Source: CAD feature listing. Evaluate the final solid. Frame: model axes, mm. A direction names the side the tool comes from. Give positions to 0.01 mm unless a question says otherwise; leave off trailing zeros. Loops run counter-clockwise (first coordinate to the right, second up) from the corner with the lowest first, then second, coordinate; pieces in that order, holes last. Notation, with made-up numbers: (-24, 88) -> (27, 88) arc R14 cw to (27, 97) -> close; hole circle Ø11 at (14, 10). An arc over 180 degrees is marked (long way). Put each result on its own line as item: value.
```python
from build123d import *

# Parameters (mm, degrees)
F0_W      = 13.86
F0_H      = 7.73
F1_DEPTH  = 2.14
F3_DEPTH  = 13.861
F4_W      = 1.7220231239
F4_H      = 4.1921688244
F5_DEPTH  = 1.48
F6_R      = 3.43
F7_DEPTH  = 1.48
F8_R      = 1.14
F10_DEPTH = 3.34
F9_R      = 1.1457110781
F11_DEPTH = 3.34
F12_R     = 1.54
F13_DEPTH = 4.39


with BuildPart() as f1:
    # F0 (on Front) → F1 (new body)
    with BuildSketch(Plane.XZ):
        with Locations((0.6576154042, 6.5625002608)):
            Rectangle(F0_W, F0_H)
    extrude(amount=F1_DEPTH)

    # F2 (on face) → F3 (cut, through all)
    with BuildSketch(Plane.YZ.offset(7.5876154042)):
        with BuildLine():
            add(Edge.make_bspline(
                [(-2.14, 4.4675002608), (-1.0178836739, 5.1285764004), (-1.0178836739, 10.7190171735), (-7.3584975292, 6.5625002608), (-3.2052818458, 3.8399072084), (-2.14, 4.4675002608)],
                knots=[0, 0, 0, 0, 0.3449820825, 0.6724910412, 1, 1, 1, 1], degree=3))
        make_face()
    extrude(amount=-F3_DEPTH, mode=Mode.SUBTRACT)

    # F4 (on Right) → F5 (join)
    with BuildSketch(Plane.YZ):
        with Locations((-2.9032976599, 6.5771206282)):
            Rectangle(F4_W, F4_H)
        Polygon((-2.042286098, 8.6732050404), (-2.042286098, 4.481036216), (-1.0486273095, 4.481036216), (-1.0486273095, 8.7523022667), align=None)
    extrude(amount=F5_DEPTH)

    # F6 (on face) → F7 (join)
    with BuildSketch(Plane.YZ.offset(1.48)):
        with Locations((-5.5470176696, 6.5771206282)):
            Circle(F6_R)
    extrude(amount=-F7_DEPTH)

    # F8 (on face) → F10 (join)
    with BuildSketch(Plane.YZ.offset(1.48)):
        with Locations((-5.5470176696, 6.5771206282)):
            Circle(F8_R)
    extrude(amount=F10_DEPTH)

    # F9 (on face) → F11 (join)
    with BuildSketch(Plane(origin=(0, 0, 0), x_dir=(0, -1, 0), z_dir=(-1, 0, 0))):
        with Locations((5.5470176696, 6.5771206282)):
            Circle(F9_R)
    extrude(amount=F11_DEPTH)

    # F12 (on face) → F13 (join)
    with BuildSketch(Plane(origin=(0, 0, 0), x_dir=(-1, 0, 0), z_dir=(0, 1, 0))):
        Polygon((-1.8146777797, 7.6139823431), (-3.245869735, 9.0531328988), (-5.2755083889, 9.0587604791), (-6.7146589446, 7.6275685238), (-6.7202865249, 5.59792987), (-5.2890945696, 4.1587793143), (-3.2594559158, 4.1531517339), (-1.8203053601, 5.5843436892), align=None)
        with Locations((-4.2674821523, 6.6059561065)):
            Circle(F12_R, mode=Mode.SUBTRACT)
        Polygon((1.7335861807, 8.9899811648), (0.294435625, 7.5587892095), (0.2888080447, 5.5291505557), (1.72, 4.09), (3.7496386538, 4.0843724197), (5.1887892095, 5.515564375), (5.2196069168, 7.5449768525), (3.7632248346, 8.9843535845), align=None)
        with Locations((2.7416124173, 6.5371767923)):
            Circle(F12_R, mode=Mode.SUBTRACT)
    extrude(amount=F13_DEPTH)


solid = f1.part
```
(1) Line query: probe 1 along Y at (x, z) = (-1.25, 6.5); probe 2 along X at (y, z) = (2.75, 7.5) (3 decimals); probe 3 along X at (y, z) = (3.5, 6.75). Output: solid intervals per line, ascending. Write a range as from..to.
Calculated:
probe 1: y = -6.69..-4.4, -1.3..0
probe 2: x = -5.219..-3.944, -1.54..-0.294, 1.815..3.014, 5.521..6.715
probe 3: x = -5.21..-4.27, -1.22..-0.29, 1.82..2.73, 5.8..6.72
(2) Reachability of faces 1 (the flat face through (0, -4, 7)), 2 (the flat face through (5.99, 2.16, 8.35)), 3 (the flat face through (6.015, 2.164, 4.888)) from +Z, -Z, +X, -X, +Y, -Y: full face, straight path, thin tool, end or side. Return the list, or none.
Calculated:
face 1: -X
face 2: +Z, +X, +Y
face 3: -Z, +X, +Y
(3) Draft query along Y for faces 4 (the flat face through (-4, 4.39, 8)), 5 (the cylindrical face through (3.44, 2.164, 7.904)), 6 (the flat face through (1.48, -4, 7)). Return one class per face: released by +Y, released by -Y, zero draft, split by the parting line, or undercut.
Calculated:
face 4: released by +Y
face 5: zero draft
face 6: undercut
(4) First-contact query: P1, Ø1.8, axis at y = -5.5, z = 7, coming from the +X side; P2, Ø3, axis at y = 2.5, z = 5.5, coming from the -X side; P3, Ø1.8, axis at x = 4.27, z = 6.61, coming from the -Y side. Flat tips, straight axial feed; report the tip coordinate or a pass-through.
Calculated:
P1: stops at x = 4.82
P2: stops at x = -5.21
P3: stops at y = -6.69
(5) Section A-A on y = 3.25. Return loops of the section in (x, z), then the cut area to 3 significant figures.
Calculated:
outline: (-5.22, 7.54) -> (-5.19, 5.52) -> (-3.75, 4.08) -> (-1.72, 4.09) -> (-0.29, 5.53) -> (-0.29, 7.56) -> (-1.73, 8.99) -> (-3.76, 8.98) -> close; (1.81, 7.61) -> (1.82, 5.58) -> (3.26, 4.15) -> (5.29, 4.16) -> (6.72, 5.6) -> (6.71, 7.63) -> (5.28, 9.06) -> (3.25, 9.05) -> close; hole circle Ø3.08 at (-2.74, 6.54); hole circle Ø3.08 at (4.27, 6.61)
area: 24.9 mm²
(6) Section B-B on z = 9.5. Return loops of the section in (x, y).
Calculated:
outline: (-6.27, -2.14) -> (7.59, -2.14) -> (7.59, 0) -> (-6.27, 0) -> close; (0, -7.34) -> (1.48, -7.34) -> (1.48, -3.75) -> (0, -3.75) -> close
(7) Section C-C on y = -7.25. Return loops of the section in (x, z), then the cut area to 3 significant figures.
Calculated:
outline: (0, 3.6) -> (1.48, 3.6) -> (1.48, 9.55) -> (0, 9.55) -> close
area: 8.81 mm²
